The listing builds one solid part. Answer for the finished solid, in the listing's coordinates (mm). A direction names the side the tool comes from. Give positions to 0.01 mm unless a question says otherwise; leave off trailing zeros. Order: outer loops, then holes, each group sorted by start corner. A loop starts at its lowest first (then second) coordinate and runs counter-clockwise, first axis right, second up. Notation, with made-up numbers: (26.5, 2.5) - (69.5, 2.5) arc R20 ccw to (69.5, 8.5) - close; hole circle Ø9 at (20.25, 37). An arc over 180 degrees is marked (long way). Answer in a Markdown table with one row per item.
from build123d import *

# Parameters (mm, degrees)
SKETCH1_R           = 3.25
SKETCH1_W           = 13.214189082
SKETCH1_H           = 8
BOSS_EXTRUDE1_DEPTH = 20


with BuildPart() as part:
    # Sketch1 → Boss-Extrude1 (new body)
    with BuildSketch(Plane.XY):
        Polygon((-8.607094541, 26.60278493), (-4.998098652, 26.60278493), (-4.998098652, 35.452037516), (4.998098652, 35.452037516), (4.998098652, 26.60278493), (8.607094541, 26.60278493), (8.607094541, 17.567007114), (3, 13.408376353), (3, -13.408376353), (8.607094541, -17.567007114), (8.607094541, -26.60278493), (4.998098652, -26.60278493), (4.998098652, -35.452037516), (-4.998098652, -35.452037516), (-4.998098652, -26.60278493), (-8.607094541, -26.60278493), (-8.607094541, -17.567007114), (-3, -13.408376353), (-3, 13.408376353), (-8.607094541, 17.567007114), align=None)
        with Locations((0, 30)):
            Circle(SKETCH1_R, mode=Mode.SUBTRACT)
        with Locations((0, -30)):
            Circle(SKETCH1_R, mode=Mode.SUBTRACT)
        with Locations((0, -20.408376353)):
            Rectangle(SKETCH1_W, SKETCH1_H, mode=Mode.SUBTRACT)
    extrude(amount=BOSS_EXTRUDE1_DEPTH)


solid = part.part
Item 1: Which of the six approach directions +Z, -Z, +X, -X, +Y, -Y give full straight-line access (tool end or side, diameter ignored) to faces 1 (the face through (5.764, -15.459, 9.86)), 2 (the face through (-7, 26.603, 10)), 3 (the face through (0, -24.408, 10)), 4 (the face through (-3, 0, 10)), 5 (the face through (-4.998, -31, 10))?
Answer block:
| item | result |
|---|---|
| face 1 | +Z, -Z, +X |
| face 2 | +Z, -Z, -X, +Y |
| face 3 | +Z, -Z |
| face 4 | +Z, -Z, -X |
| face 5 | +Z, -Z, -X, -Y |
Item 2: Each of these flat-tipped pins is pushed along its axis until it touches: P1, Ø4, axis at x = 6.5, z = 5.5, coming from the +Y side; P2, Ø7, axis at y = 33, z = 11.5, coming from the +X side; P3, Ø1.8, axis at x = -6.5, z = 8.5, coming from the +Y side; P4, Ø6, axis at y = -2.5, z = 10, coming from the -X side. Where does it stop, or does it pass through?
Answer block:
| item | result |
|---|---|
| P1 | y = 35.45 |
| P2 | x = 5 |
| P3 | y = 26.6 |
| P4 | x = -3 |
Item 3: Consider line 1 (Y direction, x = 0, z = 14.5); line 2 (Y direction, x = -1.25, z = 8.5); line 3 (Y direction, x = 4.25, z = 7.25). Determine where each line is inside the solid, lowest interval first.
Answer block:
| item | result |
|---|---|
| line 1 | -35.45 to -33.25, -26.75 to -24.41, -16.41 to 26.75, 33.25 to 35.45 |
| line 2 | -35.45 to -33, -27 to -24.41, -16.41 to 27, 33 to 35.45 |
| line 3 | -35.45 to -24.41, -16.41 to -14.34, 14.34 to 35.45 |
Item 4: Determine the mould class of faces 6 (the face through (0, -35.452, 10)), 7 (the face through (7, 26.603, 10)), 8 (the face through (6.607, -20, 10)), 9 (the face through (4.998, 31, 10)) for opening direction Y: pulls with the +Y half, pulls with the -Y half, needs draft (parallel to the pull), parting line crosses it, or undercut.
Answer block:
| item | result |
|---|---|
| face 6 | pulls with the -Y half |
| face 7 | pulls with the +Y half |
| face 8 | undercut |
| face 9 | needs draft |
Item 5: Find section B-B on y = -30. Write down the section's boundary in (x, z), then the cut area to 3 significant figures.
Answer block:
| item | result |
|---|---|
| outline | (-5, 0) - (-3.25, 0) - (-3.25, 20) - (-5, 20) - close; (3.25, 0) - (5, 0) - (5, 20) - (3.25, 20) - close |
| area | 69.9 mm² |
Item 6: Find section A-A on x = 0. Write down the section's boundary in (y, z).
Answer block:
| item | result |
|---|---|
| outline | (-35.45, 0) - (-33.25, 0) - (-33.25, 20) - (-35.45, 20) - close; (-26.75, 0) - (-24.41, 0) - (-24.41, 20) - (-26.75, 20) - close; (-16.41, 0) - (26.75, 0) - (26.75, 20) - (-16.41, 20) - close; (33.25, 0) - (35.45, 0) - (35.45, 20) - (33.25, 20) - close |
Item 7: Find section C-C on z = 9.75. Write down the section's boundary in (x, y), then the cut area to 3 significant figures.
Answer block:
| item | result |
|---|---|
| outline | (-8.61, -26.6) - (-5, -26.6) - (-5, -35.45) - (5, -35.45) - (5, -26.6) - (8.61, -26.6) - (8.61, -17.57) - (3, -13.41) - (3, 13.41) - (8.61, 17.57) - (8.61, 26.6) - (5, 26.6) - (5, 35.45) - (-5, 35.45) - (-5, 26.6) - (-8.61, 26.6) - (-8.61, 17.57) - (-3, 13.41) - (-3, -13.41) - (-8.61, -17.57) - close; hole (-6.61, -24.41) - (6.61, -24.41) - (6.61, -16.41) - (-6.61, -16.41) - close; hole circle Ø6.5 at (0, -30); hole circle Ø6.5 at (0, 30) |
| area | 573 mm² |
Item 8: Find section D-D on x = 5.75. Write down the section's boundary in (y, z).
Answer block:
| item | result |
|---|---|
| outline | (-26.6, 0) - (-24.41, 0) - (-24.41, 20) - (-26.6, 20) - close; (-16.41, 0) - (-15.45, 0) - (-15.45, 20) - (-16.41, 20) - close; (15.45, 0) - (26.6, 0) - (26.6, 20) - (15.45, 20) - close |
